Verification items for the finished model (mm, model axes). A direction names the side the tool comes from. Give positions to 0.01 mm unless a question says otherwise; leave off trailing zeros. Order: outer loops, then holes, each group sorted by start corner. A loop starts at its lowest first (then second) coordinate and runs counter-clockwise, first axis right, second up.
(1) Sectioned sample at D-D on x = -46. Record the cut outline in (y, z), plus the area to 3 significant figures.
(2) Mould release check, pull along Y, two halves, no side actions. Record for faces 3 (the face through (-69.26, 10.33, 4.93)), 4 (the face through (-72.21, 61.22, 4.93)), 5 (the face through (-66, -25.77, 5)), 6 (the face through (-67, 23, 10)): pulls with the +Y half, pulls with the -Y half, needs draft (parallel to the pull), parting line crosses it, or undercut.
(3) Scan lines: L1, parallel to X at y = -4.5, z = 6; L2, parallel to X at y = 40, z = 1.25; L3, parallel to Y at x = -57, z = 2. Record each from-to range of solid material in increasing order.
(4) Sectioned sample at A-A on y = 5. Record the cut outline in (x, z), plus the area to 3 significant figures.
(5) Gauge pin test, flat ends, axial feed: pin 1 (3 mm diameter, centred on x = -104, z = 7, fed in from -Y); pin 2 (5 mm diameter, centred on x = -105, z = 4, fed in from +Y); pin 3 (3 mm diameter, centred on x = -24.5, z = 7.5, fed in from +Y). Record the tip position at first contact, or that the pin passes through.
(6) Sectioned sample at C-C on x = -75. Record the cut outline in (y, z), plus the area to 3 significant figures.
(7) Access from +Z, -Z, +X, -X, +Y, -Y to the whole of each face (thin tool, end or side, straight path). Record for faces 1 (the face through (-92.032, 39.159, 4.93)), 2 (the face through (-67, 23, 0)).
(8) Sectioned sample at B-B on z = 3.75. Count the separate pieces of the cut face and the enclosed holes in it, plus the area to 3 significant figures.
```python
from build123d import *

# Parameters (mm, degrees)
EXTRUDE_1_DEPTH     = 10
CUT_EXTRUDE_1_DEPTH = 149.427210809
OTHER_1_DEPTH       = 10


# Read off the part's stored shape, not the designer's step: Массив, управляемый таблицей1
with BuildPart() as part:
    # Эскиз1_fr → Бобышка-Вытянуть1 (new body)
    with BuildSketch(Plane.XY):
        with BuildLine():
            Line((0, 0), (0, 20))
            add(Edge.make_bspline(
                [(0, 20), (0, 38.146025899), (-14.209474182, 48.611098897), (-41.986949672, 54.649680525)],
                knots=[0, 0, 0, 0, 1, 1, 1, 1], degree=3))
            Line((-41.986949672, 54.649680525), (-103.301225383, 67.978870897))
            add(Edge.make_bspline(
                [(-103.301225383, 67.978870897), (-115.500001367, 70.63077872), (-131.292525164, 63.393306184), (-131.292525164, 43.097715536)],
                knots=[0, 0, 0, 0, 1, 1, 1, 1], degree=3))
            Line((-131.292525164, 43.097715536), (-131.292525164, 0))
            add(Edge.make_bspline(
                [(-97.969549234, -25.769768053), (-112.011160689, -25.769768053), (-131.292525164, -19.025155818), (-131.292525164, 0)],
                knots=[0, 0, 0, 0, 1, 1, 1, 1], degree=3))
            Line((-97.969549234, -25.769768053), (-33.545129103, -25.769768053))
            add(Edge.make_bspline(
                [(-33.545129103, -25.769768053), (-19.444866568, -25.769768053), (0, -19.063757455), (0, 0)],
                knots=[0, 0, 0, 0, 1, 1, 1, 1], degree=3))
        make_face()
    extrude(amount=EXTRUDE_1_DEPTH)

    # Эскиз2_fr → Вырез-Вытянуть1 (cut, through all)
    with BuildSketch(Plane(origin=(0, 0, 0), x_dir=(-1, 0, 0), z_dir=(0, 0, -1))):
        with BuildLine():
            Line((102.429251955, 61.832882372), (104.527789693, 52.179608775))
            ThreePointArc((104.527789693, 52.179608775), (103.259303337, 50.206407776), (101.286102339, 51.474894133))
            Line((101.286102339, 51.474894133), (99.1875646, 61.128167729))
            ThreePointArc((99.1875646, 61.128167729), (100.456050956, 63.101368728), (102.429251955, 61.832882372))
        make_face()
    extrude(amount=-CUT_EXTRUDE_1_DEPTH, mode=Mode.SUBTRACT)

    # Массив, управляемый таблицей1 outline → Массив, управляемый таблицей1 (cut)
    with BuildSketch(Plane.XY):
        with BuildLine():
            ThreePointArc((-59.89006563, -3.637341625), (-61.158551986, -1.664140626), (-63.131752985, -2.932626983))
            Line((-63.131752985, -2.932626983), (-65.230290724, -12.585900579))
            ThreePointArc((-65.230290724, -12.585900579), (-63.961804368, -14.559101578), (-61.988603369, -13.290615222))
            Line((-61.988603369, -13.290615222), (-59.89006563, -3.637341625))
        make_face()
        with BuildLine():
            ThreePointArc((-68.026121008, 8.36493328), (-69.294607365, 10.338134278), (-71.267808363, 9.069647922))
            Line((-71.267808363, 9.069647922), (-73.366346102, -0.583625675))
            ThreePointArc((-73.366346102, -0.583625675), (-72.097859745, -2.556826673), (-70.124658747, -1.288340317))
            Line((-70.124658747, -1.288340317), (-68.026121008, 8.36493328))
        make_face()
        with BuildLine():
            ThreePointArc((-83.3210554, 32.157053445), (-84.589541757, 34.130254443), (-86.562742755, 32.861768087))
            Line((-86.562742755, 32.861768087), (-88.661280493, 23.208494491))
            ThreePointArc((-88.661280493, 23.208494491), (-87.392794137, 21.235293492), (-85.419593138, 22.503779848))
            Line((-85.419593138, 22.503779848), (-83.3210554, 32.157053445))
        make_face()
        with BuildLine():
            ThreePointArc((-90.968522596, 44.053113527), (-92.237008952, 46.026314526), (-94.210209951, 44.75782817))
            Line((-94.210209951, 44.75782817), (-96.308747689, 35.104554573))
            ThreePointArc((-96.308747689, 35.104554573), (-95.040261333, 33.131353574), (-93.067060334, 34.399839931))
            Line((-93.067060334, 34.399839931), (-90.968522596, 44.053113527))
        make_face()
    extrude(amount=OTHER_1_DEPTH, mode=Mode.SUBTRACT)


solid = part.part
```
Ans:
1. outline: (-25.77, 0) - (55.52, 0) - (55.52, 10) - (-25.77, 10) - close
1. area: 813 mm2
2. face 3: undercut
2. face 4: pulls with the +Y half
2. face 5: pulls with the -Y half
2. face 6: needs draft
3. L1: x = -130.91 to -63.47, -60.08 to -0.39
3. L2: x = -131.29 to -95.24, -91.85 to -8.44
3. L3: y = -25.77 to 57.91
4. outline: (-131.29, 0) - (-72.15, 0) - (-72.15, 10) - (-131.29, 10) - close; (-68.76, 0) - (0, 0) - (0, 10) - (-68.76, 10) - close
4. area: 1,280 mm2
5. pin 1: stops at y = -25.54
5. pin 2: stops at y = 68.49
5. pin 3: stops at y = 50.12
6. outline: (-25.77, 0) - (61.83, 0) - (61.83, 10) - (-25.77, 10) - close
6. area: 876 mm2
7. face 1: +Z, -Z
7. face 2: -Z, +X, -X, +Y, -Y
8. separate pieces: 1
8. enclosed holes: 5
8. area: 10,300 mm2
